Geometry check sheet. Reference: drawing and pictorial views, mm from the part's lowest x, y, z. A direction names the side the tool comes from. Give positions to 0.01 mm unless a question says otherwise; leave off trailing zeros. Write each loop counter-clockwise with the first axis right and the second up, starting at its lowest first coordinate (ties: lowest second). Pieces come first, ordered by that corner, then holes.
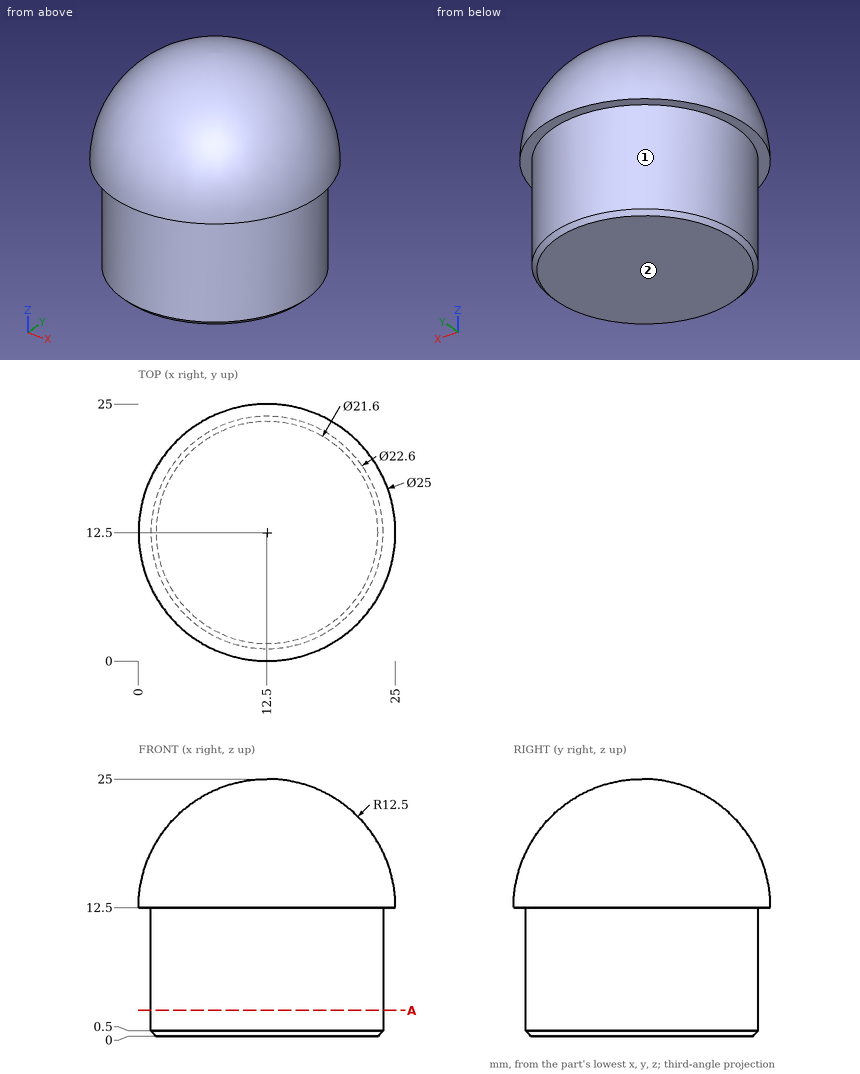
Item 1: Depth check by flat-ended pin: pin 1 (3 mm diameter, centred on x = 4, y = 3.5, fed in from +Z); pin 2 (3 mm diameter, centred on y = 3.5, z = 20.5, fed in from -X); pin 3 (6 mm diameter, centred on y = 10, z = 9, fed in from +X). Enter the tip coordinate at first touch or a pass-through.
Answer key:
pin 1: stops at z = 18.66
pin 2: stops at x = 5.78
pin 3: stops at x = 23.8
Item 2: Set-up check for the marked faces 1 and 2: record each of +Z, -Z, +X, -X, +Y, -Y from which the full face is reachable in a straight line by a thin tool's end or side.
Answer key:
face 1: -Z
face 2: -Z, +X, -X, +Y, -Y
Item 3: Sectioned sample at A-A on z = 2.5. Record the cut outline in (x, y), then the cut area to 3 significant figures.
Answer key:
outline: circle Ø22.6 at (12.5, 12.5)
area: 401 mm2
Item 4: Scan lines: line 1 along X through (y, z) = (9.5, 10.5); line 2 along Y through (x, z) = (8, 18.25); line 3 along Z through (x, y) = (19.25, 14.5). Record each from-to range of solid material in increasing order.
Answer key:
line 1: x = 1.61 to 23.39
line 2: y = 2.35 to 22.65
line 3: z = 0 to 22.83
